Can you work these out from the model? Positions are in its coordinate system, mm. Round coordinates to 2 decimals unless told otherwise and drop trailing zeros. Order: outer loops, then holes, each group sorted by start corner. A loop starts at its lowest first (then second) coordinate and runs counter-clockwise, first axis right, second up. Notation, with made-up numbers: (32, 10.5) - (43, 10.5) arc R22 cw to (43, 21.5) - close; hole circle Ø8 at (-25, -3). An arc over 180 degrees is marked (long way). Write item = value, one per line.
from build123d import *

# Parameters (mm, degrees)
F0_R     = 44.45
F0_R_2   = 1.5875
F1_DEPTH = 3.175
F2_R     = 12.7
F3_R     = 6.35


with BuildPart() as f1:
    # F0 (on Top) → F1 (new body)
    with BuildSketch(Plane.XY):
        Circle(F0_R)
        with BuildLine():
            ThreePointArc((39.2548577101, 12.7546764428), (40.7668362581, 6.4568325445), (41.275, 0))
            ThreePointArc((41.275, 0), (36.7762942859, -18.7384578767), (24.2608362884, -33.3921764428))
            ThreePointArc((24.2608362884, -33.3921764428), (0, -41.275), (-24.2608362884, -33.3921764428))
            ThreePointArc((-24.2608362884, -33.3921764428), (-39.2548577101, -12.7546764428), (-39.2548577101, 12.7546764428))
            ThreePointArc((-39.2548577101, 12.7546764428), (-24.2608362884, 33.3921764428), (0, 41.275))
            ThreePointArc((0, 41.275), (24.2608362884, 33.3921764428), (39.2548577101, 12.7546764428))
        make_face(mode=Mode.SUBTRACT)
        with BuildLine():
            Line((-1.0361992177, 38.0859067265), (0, 41.275))
            ThreePointArc((0, 41.275), (-24.2608362884, 33.3921764428), (-39.2548577101, 12.7546764428))
            Line((-39.2548577101, 12.7546764428), (-35.9016466034, 12.7546764428))
            ThreePointArc((-35.9016466034, 12.7546764428), (-22.3946181123, 30.8235474857), (-1.0361992177, 38.0859067265))
        make_face()
        with BuildLine():
            ThreePointArc((-39.2548577101, 12.7546764428), (-39.2548577101, -12.7546764428), (-24.2608362884, -33.3921764428))
            Line((-24.2608362884, -33.3921764428), (-23.2246370707, -30.2030831693))
            ThreePointArc((-23.2246370707, -30.2030831693), (-36.2352532708, -11.7735474857), (-36.5420529391, 10.7837084065))
            Line((-36.5420529391, 10.7837084065), (-39.2548577101, 12.7546764428))
        make_face()
        with BuildLine():
            ThreePointArc((-24.2608362884, -33.3921764428), (0, -41.275), (24.2608362884, -33.3921764428))
            Line((24.2608362884, -33.3921764428), (21.5480315174, -31.4212084065))
            ThreePointArc((21.5480315174, -31.4212084065), (0, -38.1), (-21.5480315174, -31.4212084065))
            Line((-21.5480315174, -31.4212084065), (-24.2608362884, -33.3921764428))
        make_face()
        with BuildLine():
            ThreePointArc((24.2608362884, -33.3921764428), (36.7762942859, -18.7384578767), (41.275, 0))
            ThreePointArc((41.275, 0), (40.7668362581, 6.4568325445), (39.2548577101, 12.7546764428))
            Line((39.2548577101, 12.7546764428), (36.5420529391, 10.7837084065))
            ThreePointArc((36.5420529391, 10.7837084065), (37.7085018065, 5.447833653), (38.1, 0))
            ThreePointArc((38.1, 0), (34.1794431815, -16.833765586), (23.2246370707, -30.2030831693))
            Line((23.2246370707, -30.2030831693), (24.2608362884, -33.3921764428))
        make_face()
        with BuildLine():
            Line((35.9016466034, 12.7546764428), (39.2548577101, 12.7546764428))
            ThreePointArc((39.2548577101, 12.7546764428), (24.2608362884, 33.3921764428), (0, 41.275))
            Line((0, 41.275), (1.0361992177, 38.0859067265))
            ThreePointArc((1.0361992177, 38.0859067265), (22.3946181123, 30.8235474857), (35.9016466034, 12.7546764428))
        make_face()
        with BuildLine():
            Line((7.7578470137, 17.398801962), (1.0361992177, 38.0859067265))
            ThreePointArc((1.0361992177, 38.0859067265), (0, 38.1), (-1.0361992177, 38.0859067265))
            Line((-1.0361992177, 38.0859067265), (-7.7578470137, 17.398801962))
            ThreePointArc((-7.7578470137, 17.398801962), (0, 19.05), (7.7578470137, 17.398801962))
        make_face()
        with BuildLine():
            Line((-14.1499374147, 12.7546764428), (-35.9016466034, 12.7546764428))
            ThreePointArc((-35.9016466034, 12.7546764428), (-36.2352532708, 11.7735474857), (-36.5420529391, 10.7837084065))
            Line((-36.5420529391, 10.7837084065), (-18.9445505487, -2.0016254668))
            ThreePointArc((-18.9445505487, -2.0016254668), (-18.1176266354, 5.8867737428), (-14.1499374147, 12.7546764428))
        make_face()
        with BuildLine():
            Line((18.9445505487, -2.0016254668), (36.5420529391, 10.7837084065))
            ThreePointArc((36.5420529391, 10.7837084065), (36.2352532708, 11.7735474857), (35.9016466034, 12.7546764428))
            Line((35.9016466034, 12.7546764428), (14.1499374147, 12.7546764428))
            ThreePointArc((14.1499374147, 12.7546764428), (17.7828401521, 6.8317710826), (19.05, 0))
            ThreePointArc((19.05, 0), (19.0236193711, -1.0022005907), (18.9445505487, -2.0016254668))
        make_face()
        with BuildLine():
            Line((3.9505291269, -18.6358745332), (21.5480315174, -31.4212084065))
            ThreePointArc((21.5480315174, -31.4212084065), (22.3946181123, -30.8235474857), (23.2246370707, -30.2030831693))
            Line((23.2246370707, -30.2030831693), (16.5029892747, -9.5159784048))
            ThreePointArc((16.5029892747, -9.5159784048), (11.1973090562, -15.4117737428), (3.9505291269, -18.6358745332))
        make_face()
        with BuildLine():
            Line((-16.5029892747, -9.5159784048), (-23.2246370707, -30.2030831693))
            ThreePointArc((-23.2246370707, -30.2030831693), (-22.3946181123, -30.8235474857), (-21.5480315174, -31.4212084065))
            Line((-21.5480315174, -31.4212084065), (-3.9505291269, -18.6358745332))
            ThreePointArc((-3.9505291269, -18.6358745332), (-11.1973090562, -15.4117737428), (-16.5029892747, -9.5159784048))
        make_face()
        with BuildLine():
            Line((-35.9016466034, 12.7546764428), (-39.2548577101, 12.7546764428))
            Line((-39.2548577101, 12.7546764428), (-36.5420529391, 10.7837084065))
            ThreePointArc((-36.5420529391, 10.7837084065), (-36.2352532708, 11.7735474857), (-35.9016466034, 12.7546764428))
        make_face()
        with BuildLine():
            Line((-23.2246370707, -30.2030831693), (-24.2608362884, -33.3921764428))
            Line((-24.2608362884, -33.3921764428), (-21.5480315174, -31.4212084065))
            ThreePointArc((-21.5480315174, -31.4212084065), (-22.3946181123, -30.8235474857), (-23.2246370707, -30.2030831693))
        make_face()
        with BuildLine():
            Line((21.5480315174, -31.4212084065), (24.2608362884, -33.3921764428))
            Line((24.2608362884, -33.3921764428), (23.2246370707, -30.2030831693))
            ThreePointArc((23.2246370707, -30.2030831693), (22.3946181123, -30.8235474857), (21.5480315174, -31.4212084065))
        make_face()
        with BuildLine():
            Line((36.5420529391, 10.7837084065), (39.2548577101, 12.7546764428))
            Line((39.2548577101, 12.7546764428), (35.9016466034, 12.7546764428))
            ThreePointArc((35.9016466034, 12.7546764428), (36.2352532708, 11.7735474857), (36.5420529391, 10.7837084065))
        make_face()
        with BuildLine():
            Line((1.0361992177, 38.0859067265), (0, 41.275))
            Line((0, 41.275), (-1.0361992177, 38.0859067265))
            ThreePointArc((-1.0361992177, 38.0859067265), (0, 38.1), (1.0361992177, 38.0859067265))
        make_face()
        with BuildLine():
            ThreePointArc((16.5029892747, -9.5159784048), (18.1176266354, -5.8867737428), (18.9445505487, -2.0016254668))
            ThreePointArc((18.9445505487, -2.0016254668), (19.0236193711, -1.0022005907), (19.05, 0))
            ThreePointArc((19.05, 0), (17.7828401521, 6.8317710826), (14.1499374147, 12.7546764428))
            ThreePointArc((14.1499374147, 12.7546764428), (11.1973090562, 15.4117737428), (7.7578470137, 17.398801962))
            ThreePointArc((7.7578470137, 17.398801962), (0, 19.05), (-7.7578470137, 17.398801962))
            ThreePointArc((-7.7578470137, 17.398801962), (-11.1973090562, 15.4117737428), (-14.1499374147, 12.7546764428))
            ThreePointArc((-14.1499374147, 12.7546764428), (-18.1176266354, 5.8867737428), (-18.9445505487, -2.0016254668))
            ThreePointArc((-18.9445505487, -2.0016254668), (-18.1176266354, -5.8867737428), (-16.5029892747, -9.5159784048))
            ThreePointArc((-16.5029892747, -9.5159784048), (-11.1973090562, -15.4117737428), (-3.9505291269, -18.6358745332))
            ThreePointArc((-3.9505291269, -18.6358745332), (0, -19.05), (3.9505291269, -18.6358745332))
            ThreePointArc((3.9505291269, -18.6358745332), (11.1973090562, -15.4117737428), (16.5029892747, -9.5159784048))
        make_face()
        Circle(F0_R_2, mode=Mode.SUBTRACT)
    extrude(amount=F1_DEPTH)

    # F2
    f2_edges = [f1.edges().sort_by_distance(p)[0] for p in [
        (-7.757847, 17.398802, 1.5875),
        (7.757847, 17.398802, 1.5875),
        (16.502989, -9.515978, 1.5875),
        (18.944551, -2.001625, 1.5875),
        (14.149937, 12.754676, 1.5875),
        (-14.149937, 12.754676, 1.5875),
        (-16.502989, -9.515978, 1.5875),
        (-18.944551, -2.001625, 1.5875),
        (-3.950529, -18.635875, 1.5875),
        (3.950529, -18.635875, 1.5875),
    ]]
    fillet(f2_edges, radius=F2_R)

    # F3
    f3_edges = [f1.edges().sort_by_distance(p)[0] for p in [
        (-21.548032, -31.421208, 1.5875),
        (21.548032, -31.421208, 1.5875),
        (-36.542053, 10.783708, 1.5875),
        (-23.224637, -30.203083, 1.5875),
        (-35.901647, 12.754676, 1.5875),
        (1.036199, 38.085907, 1.5875),
        (23.224637, -30.203083, 1.5875),
        (-1.036199, 38.085907, 1.5875),
        (35.901647, 12.754676, 1.5875),
        (36.542053, 10.783708, 1.5875),
    ]]
    fillet(f3_edges, radius=F3_R)


solid = f1.part
(1) If I drill on line 1 (Y direction, x = 0, z = 1.75); line 2 (Y direction, x = 25.5, z = 2); line 3 (X direction, y = -7.5, z = 0.6), over which ranges is the centre line in solid material (lowest first)? Write a range as from..to.
Computed:
line_1 = -44.45..-38.1, -19.05..-1.59, 1.59..44.45
line_2 = -36.41..-24.54, 2.76..12.76, 28.31..36.41
line_3 = -43.81..-37.35, -17.66..17.66, 37.35..43.81
(2) Will these pins go through, and if not, where does the flat tip stop? P1, Ø5, axis at x = 0, y = 0, coming from the +Z side (3 decimals); P2, Ø1, axis at y = -23.5, z = 1, coming from the -X side; P3, Ø1, axis at x = 22.5, z = 2, coming from the +Y side; P4, Ø1.6, axis at x = -23.5, z = 1.5, coming from the +Y side.
Computed:
P1 = 3.175
P2 = -38.04
P3 = 38.62
P4 = 38.22
(3) If we section it at C-C (y = 26): Write out the boundary of the cut face in (x, z) (3 decimals), plus the area to 3 significant figures.
Computed:
outline = (-36.053, 0) - (-27.85, 0) - (-27.85, 3.175) - (-36.053, 3.175) - close; (-4.963, 0) - (4.963, 0) - (4.963, 3.175) - (-4.963, 3.175) - close; (27.85, 0) - (36.053, 0) - (36.053, 3.175) - (27.85, 3.175) - close
area = 83.6 mm^2
(4) If we section it at A-A (y = -17.5): Write out the boundary of the cut face in (x, z) (3 decimals), plus the area to 3 significant figures.
Computed:
outline = (-40.86, 0) - (-33.843, 0) - (-33.843, 3.175) - (-40.86, 3.175) - close; (-19.097, 0) - (19.097, 0) - (19.097, 3.175) - (-19.097, 3.175) - close; (33.843, 0) - (40.86, 0) - (40.86, 3.175) - (33.843, 3.175) - close
area = 166 mm^2
(5) If we section it at B-B (z = 0.9): State how many separate pieces and enclosed holes the cut face has, plus the area to 3 significant figures.
Computed:
separate_pieces = 1
enclosed_holes = 6
area = 3,910 mm^2
